Design review of the part built by this model. Coordinates are the model's own, in mm. Face numbers are marked on the shaded views. A direction names the side the tool comes from. Round coordinates to 2 decimals unless told otherwise and drop trailing zeros. Order: outer loops, then holes, each group sorted by start corner. A loop starts at its lowest first (then second) coordinate and runs counter-clockwise, first axis right, second up.
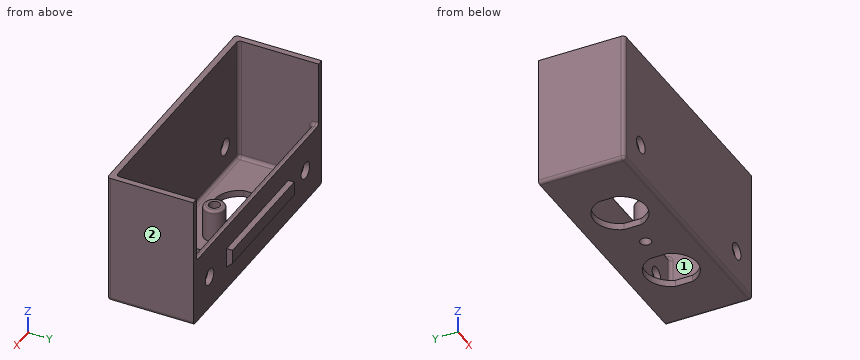
from build123d import *

# Parameters (mm, degrees)
F0_W      = 75
F0_H      = 26
F1_DEPTH  = 2
F2_W      = 75
F2_H      = 26
F2_W_2    = 71.4
F2_H_2    = 22.4
F3_DEPTH  = 38
F5_DEPTH  = 2
F6_R      = 2.5
F7_DEPTH  = 1.8
F8_W      = 36
F8_H      = 6
F9_DEPTH  = 1.8
F10_SIZE  = 1.79999
F11_W     = 71.4
F11_H     = 1.8
F12_DEPTH = 20
F13_R     = 3.125
F14_DEPTH = 10
F15_R     = 0.75
F16_R     = 1.65
F17_DEPTH = 40.001
F18_F1_R  = 1
F18_F2_R  = 1
F19_R     = 2.5
F20_DEPTH = 27.801


# Not quite as in the source:
# - a fillet or chamfer is up to 0.001 mm smaller than in the source, because OpenCascade refuses the exact size


with BuildPart() as f1:
    # F0 (on Top) → F1 (new body)
    with BuildSketch(Plane.XY):
        Rectangle(F0_W, F0_H)
    extrude(amount=F1_DEPTH)

    # F2 (on face) → F3 (join)
    with BuildSketch(Plane.XY.offset(2)):
        Rectangle(F2_W, F2_H)
        Rectangle(F2_W_2, F2_H_2, mode=Mode.SUBTRACT)
    extrude(amount=F3_DEPTH)

    # F4 (on face) → F5 (cut, through all)
    with BuildSketch(Plane(origin=(0, 0, 0), x_dir=(1, 0, 0), z_dir=(0, 0, -1))):
        with BuildLine():
            Line((-22.35, 2.6110342778), (-22.35, -2.6110342778))
            ThreePointArc((-22.35, -2.6110342778), (-15, -7.8), (-7.65, -2.6110342778))
            Line((-7.65, -2.6110342778), (-7.65, 2.6110342778))
            ThreePointArc((-7.65, 2.6110342778), (-15, 7.8), (-22.35, 2.6110342778))
        make_face()
        with BuildLine():
            ThreePointArc((22.35, 2.6110342778), (15, 7.8), (7.65, 2.6110342778))
            Line((7.65, 2.6110342778), (7.65, -2.6110342778))
            ThreePointArc((7.65, -2.6110342778), (15, -7.8), (22.35, -2.6110342778))
            Line((22.35, -2.6110342778), (22.35, 2.6110342778))
        make_face()
    extrude(amount=-F5_DEPTH, mode=Mode.SUBTRACT)

    # F6 (on face) → F7 (cut, through all)
    with BuildSketch(Plane(origin=(0, 13, 0), x_dir=(-1, 0, 0), z_dir=(0, 1, 0))):
        with Locations((28, 10)):
            Circle(F6_R)
        with Locations((-28, 10)):
            Circle(F6_R)
    extrude(amount=-F7_DEPTH, mode=Mode.SUBTRACT)

    # F8 (on face) → F9 (join)
    with BuildSketch(Plane(origin=(0, 13, 0), x_dir=(-1, 0, 0), z_dir=(0, 1, 0))):
        with Locations((0, 10)):
            Rectangle(F8_W, F8_H)
    extrude(amount=F9_DEPTH)

    # F10 (size 1.8 in the source; OpenCascade refuses exactly that, so slightly less here)
    f10_edges = [f1.edges().sort_by_distance(p)[0] for p in [
        (0, 14.8, 7),
    ]]
    chamfer(f10_edges, length=F10_SIZE)

    # F11 (on face) → F12 (cut)
    with BuildSketch(Plane.XY.offset(40)):
        with Locations((0, 12.1)):
            Rectangle(F11_W, F11_H)
    extrude(amount=-F12_DEPTH, mode=Mode.SUBTRACT)

    # F13 (on face) → F14 (join)
    with BuildSketch(Plane.XY.offset(2)):
        Circle(F13_R)
    extrude(amount=F14_DEPTH)

    # F15
    f15_edges = [f1.edges().sort_by_distance(p)[0] for p in [
        (-3.125, 0, 12),
    ]]
    fillet(f15_edges, radius=F15_R)

    # F16 (on face) → F17 (cut, through all)
    with BuildSketch(Plane(origin=(0, 0, 0), x_dir=(1, 0, 0), z_dir=(0, 0, -1))):
        Circle(F16_R)
    extrude(amount=-F17_DEPTH, mode=Mode.SUBTRACT)

    # F18: fillet of radius 1 on 14 edges, made by hand

    # F18_f1
    f18_f1_edges = [f1.edges().sort_by_distance(p)[0] for p in [
        (-37.5, -13, 20),
        (37.5, -13, 20),
        (0, -13, 0),
        (37.5, 0, 0),
        (-37.5, 0, 0),
        (0, 11.2, 20),
    ]]
    fillet(f18_f1_edges, radius=F18_F1_R)

    # F18_f2
    f18_f2_edges = [f1.edges().sort_by_distance(p)[0] for p in [
        (-35.7, -11.2, 21),
        (35.7, -11.2, 21),
        (0, -11.2, 2),
        (35.7, 0, 2),
        (-35.7, 0, 2),
        (0, 11.2, 2),
        (35.7, 11.2, 10.5),
        (-35.7, 11.2, 10.5),
        (-35.7, 11.4928932188, 19.7071067812),
        (35.7, 11.4928932188, 19.7071067812),
    ]]
    fillet(f18_f2_edges, radius=F18_F2_R)

    # F19 (on face) → F20 (cut, through all)
    with BuildSketch(Plane.XZ.offset(13)):
        with Locations((28, 10)):
            Circle(F19_R)
        with Locations((-28, 10)):
            Circle(F19_R)
    extrude(amount=-F20_DEPTH, mode=Mode.SUBTRACT)


solid = f1.part
1) Take a section at A-A on y = 0. State how many separate pieces and enclosed holes the cut face has, plus the area to 3 significant figures.
Results:
separate pieces: 4
enclosed holes: 0
area: 251 mm2
2) To check wall thickness, follow line 1 along X through (y, z) = (12.1, 10); line 2 along X through (y, z) = (1.5, 20.5); line 3 along Y through (x, z) = (-5, 3.5). State the ranges of each line that lie inside material, in increasing order.
Results:
line 1: x = -37.5 to -30.5, -25.5 to 25.5, 30.5 to 37.5
line 2: x = -37.5 to -35.7, 35.7 to 37.5
line 3: y = -13 to -11.2, 11.2 to 13
3) For the marked faces 1 and 2, list the 3-axis set-ups (+Z, -Z, +X, -X, +Y, -Y) from which the entire face can be reached by the end or side of a thin tool; tool diameter is ignored.
Results:
face 1: +Z
face 2: +Z, -Z, +X, +Y, -Y
4) Clearance check with flat-ended pins moving along their axes: P1, Ø0.9, axis at x = 12.5, y = 13, coming from the +Z side; P2, Ø5, axis at x = -26.5, z = 4.5, coming from the +Y side; P3, Ø4, axis at x = 0, y = 0, coming from the +Z side. State where each tip first meets the part, or that it passes through.
Results:
P1: stops at z = 20
P2: stops at y = 13
P3: stops at z = 12
5) Take a section at C-C on x = -28. Give the boundary of the cut face in (y, z).
Results:
outline: (-13, 1) arc R1 ccw to (-12, 0) - (13, 0) - (13, 7.5) - (11.2, 7.5) - (11.2, 3) arc R1 cw to (10.2, 2) - (-10.2, 2) arc R1 cw to (-11.2, 3) - (-11.2, 7.5) - (-13, 7.5) - close; (-13, 12.5) - (-11.2, 12.5) - (-11.2, 40) - (-13, 40) - close; (11.2, 12.5) - (13, 12.5) - (13, 20) - (12.2, 20) arc R1 ccw to (11.2, 19) - close
